from build123d import *

# Parameters (mm, degrees)
SKETCH_1_R          = 50
EXTRUDE_1_DEPTH     = 100
SKETCH_2_R          = 6.693038614
CUT_EXTRUDE_1_DEPTH = 5


with BuildPart() as part:
    # 草图1 → 凸台-拉伸1 (new body)
    with BuildSketch(Plane.XY):
        with BuildLine():
            Line((-51.262135922, 98.058252427), (-51.262135922, -101.941747573))
            Line((-51.262135922, -101.941747573), (68.737864078, -101.941747573))
            Line((68.737864078, -101.941747573), (68.737864078, 98.058252427))
            ThreePointArc((68.737864078, 98.058252427), (8.737864078, 158.058252427), (-51.262135922, 98.058252427))
        make_face()
        with Locations((8.737864078, 98.058252427)):
            Circle(SKETCH_1_R, mode=Mode.SUBTRACT)
    extrude(amount=EXTRUDE_1_DEPTH)

    # 草图2 → 切除-拉伸1 (cut)
    with BuildSketch(Plane(origin=(0, -101.941747573, 0), x_dir=(-1, 0, 0), z_dir=(0, -1, 0))):
        with Locations(Location((-8.737864078, -52.248339219, 0), (0, 0, 90))):
            Circle(SKETCH_2_R)
    extrude(amount=-CUT_EXTRUDE_1_DEPTH, mode=Mode.SUBTRACT)


solid = part.part
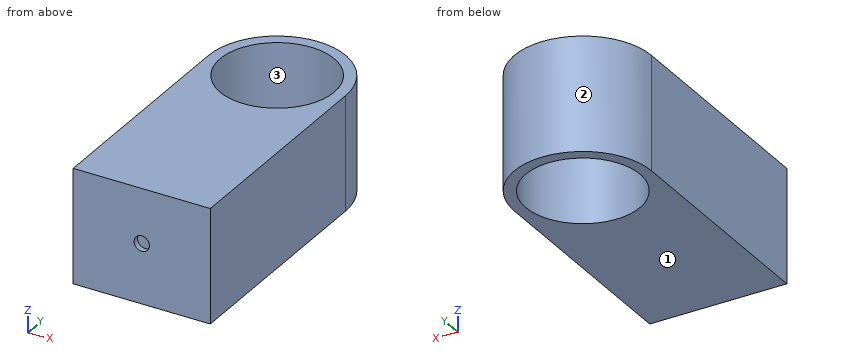
The model under review builds one solid part; all positions refer to its coordinate system, in mm. Face numbers are marked on the shaded views. Coordinates: 2 decimals unless noted, no trailing zeros. Loops run counter-clockwise (first coordinate to the right, second up) from the corner with the lowest first, then second, coordinate; pieces in that order, holes last. Notation, with made-up numbers: (-1, -35.75) -> (24, -35.75) arc R27 cw to (24, 1.25) -> close; hole circle Ø3 at (22, 6). An arc over 180 degrees is marked (long way). Use a Markdown table: item, result. Add a question column.
1. Add section B-B on x = -1.5. Write out the cut boundary in (y, z), plus the area to 3 significant figures.
2. Draft analysis for pull direction X (two halves, no side actions). For the marked faces 1, 2 and 3, state which applies: pulls with the +X half, pulls with the -X half, needs draft (parallel to the pull), parting line crosses it, or undercut.
3. Add section A-A on y = 73. Write out the cut boundary in (x, z), plus the area to 3 significant figures.
4. Clearance check with flat-ended pins moving along their axes: pin 1 Ø8 at (x, z) = (8.74, 52.25) entering from +Y; pin 2 Ø8 at (x, z) = (37.5, 61) entering from +Y; pin 3 Ø4 at (y, z) = (102, 16.5) entering from -X. State where each tip first meets the part, or that it passes through.
5. Add section C-C on z = 27. Write out the cut boundary in (x, y).
6. To check wall thickness, follow line 1 (Y direction, x = 9, z = 73); line 2 (X direction, y = 89, z = 75.5); line 3 (Y direction, x = 21, z = 94). State the ranges of each line that lie inside material, in increasing order.
Returned:
| question | item | result |
|---|---|---|
| 1 | outline | (-101.94, 0) -> (49.12, 0) -> (49.12, 100) -> (-101.94, 100) -> close; (147, 0) -> (157.18, 0) -> (157.18, 100) -> (147, 100) -> close |
| 1 | area | 16,100 mm² |
| 2 | face 1 | needs draft |
| 2 | face 2 | parting line crosses it |
| 2 | face 3 | undercut |
| 3 | outline | (-51.26, 0) -> (-34.53, 0) -> (-34.53, 100) -> (-51.26, 100) -> close; (52.01, 0) -> (68.74, 0) -> (68.74, 100) -> (52.01, 100) -> close |
| 3 | area | 3,350 mm² |
| 4 | pin 1 | stops at y = 158.06 |
| 4 | pin 2 | stops at y = 152.71 |
| 4 | pin 3 | stops at x = -51.23 |
| 5 | outline | (-51.26, -101.94) -> (68.74, -101.94) -> (68.74, 98.06) arc R60 ccw to (-51.26, 98.06) -> close; hole circle Ø100 at (8.74, 98.06) |
| 6 | line 1 | y = -101.94 to 48.06, 148.06 to 158.06 |
| 6 | line 2 | x = -51.26 to -40.43, 57.91 to 68.74 |
| 6 | line 3 | y = -101.94 to 49.59, 146.53 to 156.79 |
